Part print with two shaded views. Sizes in mm from the minimum x, y, z corner. Give positions to 0.01 mm unless a question says otherwise; leave off trailing zeros. Write each loop counter-clockwise with the first axis right and the second up, starting at its lowest first coordinate (ties: lowest second). Pieces come first, ordered by that corner, then holes. Notation, with made-up numbers: (60.5, 72) -> (117.5, 72) arc R20 cw to (117.5, 108) -> close; hole circle Ø1 at (53, -3). An arc over 180 degrees is marked (long way). Write item = value, one per line. Start each with the question number.
Q1. Wall check: line 1 (Z direction, x = 4, y = 0.75) (3 decimals); line 2 (Z direction, x = 36, y = 0.8). Give the ranges that are in metal, low to high.
Q2. Saw through at B-B, the plane x = 4. List the corners of the cut face in (y, z) (3 decimals).
Q3. Saw through at A-A, the plane y = 1. List the corners of the cut face in (x, z) (3 decimals), then the cut area to 3 significant figures.
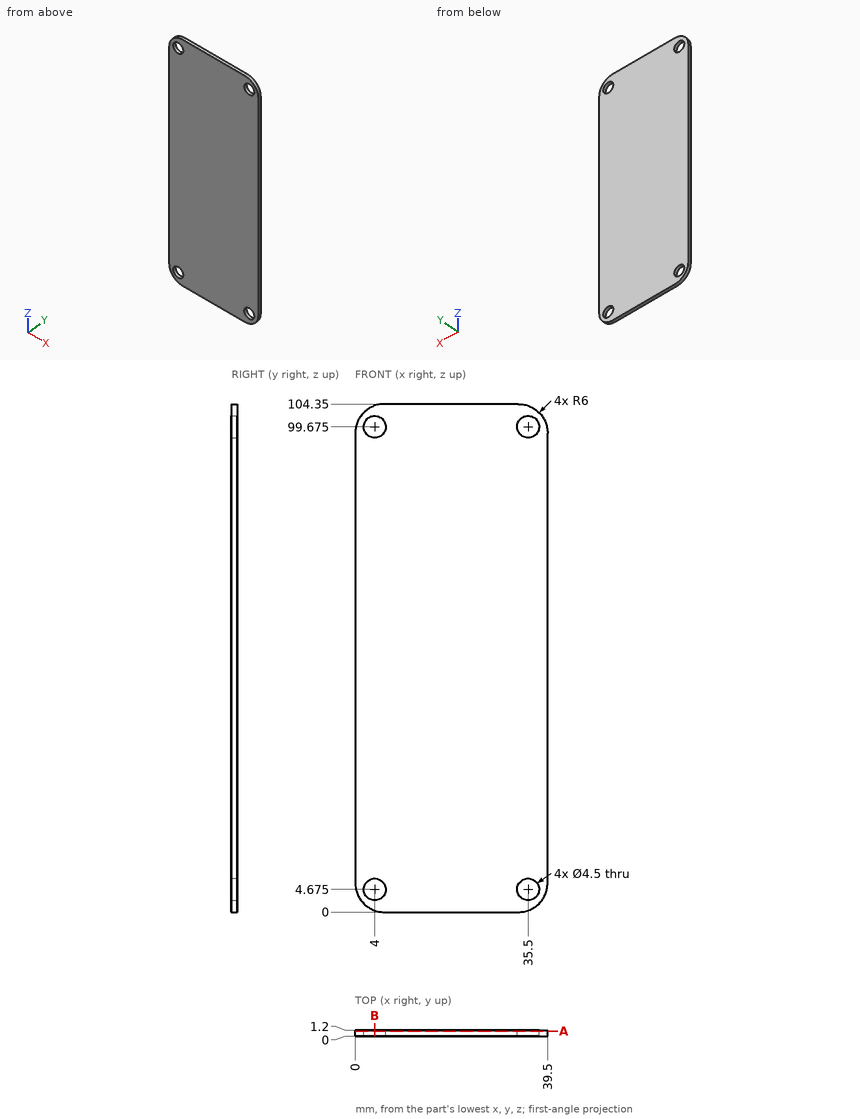
Report:
q1.line_1 = 0.343 to 2.425, 6.925 to 97.425, 101.925 to 104.007
q1.line_2 = 0.55 to 2.48, 6.87 to 97.48, 101.87 to 103.8
q2.outline = (0, 0.343) -> (1.2, 0.343) -> (1.2, 2.425) -> (0, 2.425) -> close; (0, 6.925) -> (1.2, 6.925) -> (1.2, 97.425) -> (0, 97.425) -> close; (0, 101.925) -> (1.2, 101.925) -> (1.2, 104.007) -> (0, 104.007) -> close
q3.outline = (0, 6) arc R6 ccw to (6, 0) -> (33.5, 0) arc R6 ccw to (39.5, 6) -> (39.5, 98.35) arc R6 ccw to (33.5, 104.35) -> (6, 104.35) arc R6 ccw to (0, 98.35) -> close; hole circle Ø4.5 at (4, 4.675); hole circle Ø4.5 at (4, 99.675); hole circle Ø4.5 at (35.5, 4.675); hole circle Ø4.5 at (35.5, 99.675)
q3.area = 4,030 mm2
